Check sheet for the modelled part. Datum: model origin and axes. Units: mm. A direction names the side the tool comes from. Round coordinates to 2 decimals unless told otherwise and drop trailing zeros. Loops run counter-clockwise (first coordinate to the right, second up) from the corner with the lowest first, then second, coordinate; pieces in that order, holes last. Notation, with made-up numbers: (29, 61) - (41, 61) arc R23 cw to (41, 89) - close; hole circle Ø6 at (-40, 40.25). An arc over 180 degrees is marked (long way). Return JSON: item names as keys, results as strings.
from build123d import *

# Parameters (mm, degrees)
SKETCH2_R          = 1.355
CUT_EXTRUDE1_DEPTH = 12.7
CIRPATTERN1_COUNT  = 4
SKETCH3_W          = 5.14577381
SKETCH3_H          = 8
EXTRUDE1_DEPTH     = 12.7
FILLET1_R          = 9.448
CUT_EXTRUDE2_REACH = 24.907
SKETCH4_W          = 10
SKETCH4_H          = 1
CUT_EXTRUDE3_DEPTH = 6
SKETCH6_R          = 1.85
CUT_EXTRUDE4_DEPTH = 3.5
CUT_EXTRUDE5_REACH = 22.487
SKETCH7_R          = 1.3525


with BuildPart() as part:
    # Sketch1 → Revolve1 (revolve)
    with BuildSketch(Plane.XY, mode=Mode.PRIVATE) as revolve1_sk:
        Polygon((5.7, 0), (8, 0), (8, 6), (11.1, 6), (11.1, -6.7), (5.7, -6.7), align=None)
    revolve(revolve1_sk.sketch.rotate(Axis((0, 9.388395062, 0), (0, -1, 0)), 90), axis=Axis((0, 9.388395062, 0), (0, -1, 0)))

    # Sketch2 → Cut-Extrude1 (cut)
    with BuildSketch(Plane(origin=(0, 6, 0), x_dir=(1, 0, 0), z_dir=(0, 1, 0))):
        with Locations(Location((5.66, 5.653706749, 0), (0, 0, 270))):
            Circle(SKETCH2_R)
    cut_extrude1 = extrude(amount=-CUT_EXTRUDE1_DEPTH, mode=Mode.SUBTRACT)

    # CirPattern1: Cut-Extrude1 ×4 about axis
    cirpattern1_axis = Axis((0, 0, 0), (0, 1, 0))
    for i in range(1, CIRPATTERN1_COUNT):
        add(cut_extrude1.rotate(cirpattern1_axis, i * 360 / CIRPATTERN1_COUNT), mode=Mode.SUBTRACT)

    # Sketch3 → Extrude1 (add)
    with BuildSketch(Plane(origin=(0, 6, 0), x_dir=(1, 0, 0), z_dir=(0, 1, 0))):
        with Locations((-12.927113095, 0)):
            Rectangle(SKETCH3_W, SKETCH3_H)
    extrude(amount=-EXTRUDE1_DEPTH)

    # Fillet1
    # the kernel refuses this fillet: 9.448 mm, written as the material it adds along each edge
    with BuildSketch(Plane(origin=(-10.35422619, 6, -4), x_dir=(-1, 0, 0), z_dir=(0, -1, 0))) as fillet1_piece_1_section:
        with BuildLine():
            CenterArc((5.181912326, 9.448), FILLET1_R, 220.879291984, 49.120708016)
            ThreePointArc((-1.961626544, 3.264590228), (-0.839750005, 1.717057191), (0, 0))
            Line((0, 0), (5.181912326, 0))
        make_face()
    fillet1_piece_1 = extrude(amount=12.7, mode=Mode.PRIVATE)
    fillet1_piece_1 = split(fillet1_piece_1, bisect_by=Plane(origin=(-15.5, -0.35, -4.693597662), z_dir=(1, 0, 0)), keep=Keep.TOP, mode=Mode.PRIVATE)
    add(fillet1_piece_1)
    with BuildSketch(Plane(origin=(-10.35422619, 6, 4), x_dir=(-1, 0, 0), z_dir=(0, -1, 0))) as fillet1_piece_2_section:
        with BuildLine():
            CenterArc((5.181912326, -9.448), FILLET1_R, 90, 49.120708016)
            ThreePointArc((-1.961626544, -3.264590228), (-0.839750005, -1.717057191), (0, 0))
            Line((0, 0), (5.181912326, 0))
        make_face()
    fillet1_piece_2 = extrude(amount=12.7, mode=Mode.PRIVATE)
    fillet1_piece_2 = split(fillet1_piece_2, bisect_by=Plane(origin=(-15.5, -0.35, 4.693597662), z_dir=(1, 0, 0)), keep=Keep.TOP, mode=Mode.PRIVATE)
    add(fillet1_piece_2)

    # Cut-Extrude2: up to this face of the body (flat: up to its plane)
    cut_extrude2_end = Plane(part.part.faces().sort_by_distance((-15.153532108, -6.7, 0))[0])
    # Sketch4 → Cut-Extrude2 (cut, up to the picked face)
    with BuildSketch(Plane(origin=(0, 6, 0), x_dir=(1, 0, 0), z_dir=(0, 1, 0)), mode=Mode.PRIVATE) as cut_extrude2_sk1:
        with Locations((-10.5, 0)):
            Rectangle(SKETCH4_W, SKETCH4_H)
    cut_extrude2_tool1 = split(extrude(cut_extrude2_sk1.sketch, amount=-CUT_EXTRUDE2_REACH, mode=Mode.PRIVATE), bisect_by=cut_extrude2_end, keep=Keep.BOTH, mode=Mode.PRIVATE)
    add(cut_extrude2_tool1.solids().sort_by(Axis((-10.5, 6, 0), (0, -1, 0)))[0], mode=Mode.SUBTRACT)

    # Sketch5 → Cut-Extrude3 (cut)
    with BuildSketch(Plane.ZY.offset(15.5)):
        with BuildLine():
            Line((4, 5.8), (4, -0.83286788))
            ThreePointArc((4, -0.83286788), (6.82068013, 2.48356606), (4, 5.8))
        make_face()
    extrude(amount=-CUT_EXTRUDE3_DEPTH, mode=Mode.SUBTRACT)

    # Sketch6 → Cut-Extrude4 (cut)
    with BuildSketch(Plane.XY.offset(4)):
        with Locations((-13, 2.48356606)):
            Circle(SKETCH6_R)
    extrude(amount=-CUT_EXTRUDE4_DEPTH, mode=Mode.SUBTRACT)

    # Sketch7 → Cut-Extrude5 (cut, up to next)
    with BuildSketch(Plane.XY.offset(-0.5), mode=Mode.PRIVATE) as cut_extrude5_sk1:
        with Locations((-13, 2.48356606)):
            Circle(SKETCH7_R)
    cut_extrude5_tool1 = extrude(cut_extrude5_sk1.sketch, amount=-CUT_EXTRUDE5_REACH, mode=Mode.PRIVATE) & part.part
    add(cut_extrude5_tool1.solids().sort_by_distance((-13, 2.483566, -0.5))[0], mode=Mode.SUBTRACT)


solid = part.part
Q1. Sectioned sample at C-C (z = -3). Enter the section's corners in (x, y) (1 decimal), plus the area to 3 significant figures.
Answer key:
{"outline": "(-15.5, -6.7) - (-4.8, -6.7) - (-4.8, 0) - (-7.4, 0) - (-7.4, 6) - (-15.5, 6) - close; (4.8, -6.7) - (10.7, -6.7) - (10.7, 6) - (7.4, 6) - (7.4, 0) - (4.8, 0) - close; hole circle Ø2.7 at (-13, 2.5)", "area": "173 mm²"}
Q2. Sectioned sample at A-A (x = 0). Enter the section's corners in (y, z), plus the area to 3 significant figures.
Answer key:
{"outline": "(-6.7, -11.1) - (6, -11.1) - (6, -8) - (0, -8) - (0, -5.7) - (-6.7, -5.7) - close; (-6.7, 5.7) - (0, 5.7) - (0, 8) - (6, 8) - (6, 11.1) - (-6.7, 11.1) - close", "area": "110 mm²"}
Q3. Sectioned sample at B-B (y = -1.5). Enter the section's corners in (x, z) (3 decimals).
Answer key:
{"outline": "(-15.5, -4) arc R9.448 cw to (-8.393, -7.265) arc R11.1 ccw (long way) to (-8.393, 7.265) arc R9.448 cw to (-15.5, 4) - (-15.5, 0.5) - (-5.678, 0.5) arc R5.7 cw (long way) to (-5.678, -0.5) - (-15.5, -0.5) - close; hole circle Ø2.71 at (-5.66, 5.654); hole circle Ø2.71 at (-5.654, -5.66); hole circle Ø2.71 at (5.654, 5.66); hole circle Ø2.71 at (5.66, -5.654)"}
Q4. Depth check by flat-ended pin: P1, Ø1.8, axis at x = -12.5, y = 2.5, coming from the +Z side; P2, Ø2.5, axis at x = 5.66, z = -5.65, coming from the +Y side; P3, Ø3, axis at x = -8.5, y = 0, coming from the +Z side; P4, Ø8, axis at x = 1, z = 3, coming from the +Y side. Enter the tip coordinate at first touch or a pass-through.
Answer key:
{"P1": "stops at z = -0.5", "P2": "passes through", "P3": "stops at z = 8.61", "P4": "stops at y = 0"}
Q5. Scan lines: probe 1 along Z at (x, y) = (0, -3.5); probe 2 along Y at (x, z) = (-13, -2.65); probe 3 along X at (y, z) = (-0.25, 6). Record each from-to range of solid material in increasing order. Write a range as [from, to].
Answer key:
{"probe 1": "z = [-11.1, -5.7], [5.7, 11.1]", "probe 2": "y = [-6.7, 1.13], [3.84, 6]", "probe 3": "x = [-9.72, -6.97], [-4.35, 4.34], [6.97, 9.34]"}
Q6. Sectioned sample at D-D (x = -13). Enter the section's corners in (y, z).
Answer key:
{"outline": "(-6.7, -4.35) - (1.13, -4.35) - (1.13, -0.5) - (-6.7, -0.5) - close; (-6.7, 0.5) - (0.63, 0.5) - (0.63, 4) - (-0.83, 4) arc R3.36 cw to (-0.76, 4.35) - (-6.7, 4.35) - close; (3.84, -4.35) - (6, -4.35) - (6, -0.5) - (3.84, -0.5) - close; (4.33, 0.5) - (6, 0.5) - (6, 4.35) - (5.72, 4.35) arc R3.36 cw to (5.8, 4) - (4.33, 4) - close"}
Q7. Tool access check on faces 4 (the face through (-11, -2, 0.5)), 5 (the face through (8, 3, 0)), 6 (the face through (-11.29, 1.78, 2.27)). Record the directions out of +Z, -Z, +X, -X, +Y, -Y that give a thin tool (end or side, any length) a straight path to the whole face; none if there is none.
Answer key:
{"face 4": "-X, +Y, -Y", "face 5": "+Y", "face 6": "+Z"}
Q8. Draft check along Z on faces 1 (the face through (5.695, -3.303, -0.244)), 2 (the face through (11.094, -0.439, -0.377)), 3 (the face through (-15.5, 0, -2)). Enter one of: released by +Z, released by -Z, zero draft, split by the parting line, or undercut.
Answer key:
{"face 1": "undercut", "face 2": "split by the parting line", "face 3": "zero draft"}
